Autodesk Inventor part; units mm, degrees
ref_plane "YZ Plane" through (0, 0, 0) normal (1, 0, 0) x (0, 1, 0)
ref_plane "XZ Plane" through (0, 0, 0) normal (0, 1, 0) x (-1, 0, 0)
ref_plane "XY Plane" through (0, 0, 0) normal (0, 0, 1) x (1, 0, 0)
sketch "Sketch3" plane through (0, 0, 0) normal (0, 1, 0) x (-1, 0, 0)
  circle A0 centre (0, 0) radius 5
  dimension "d8" = 10
extrude "Extrusion3" add sketch "Sketch3" along normal blind 20
sketch "Sketch4" plane through (0, 0, 0) normal (1, 0, 0) x (0, 1, 0)
  circle A0 centre (25, 0) radius 3.5
  circle A1 centre (25, 0) radius 5
  line L0 (20, -5) -> (20, 5)
  line L1 (20, -5) -> (25, -5)
  line L2 (20, 5) -> (25, 5)
  point P0 (0, 0)
  point P1 (25, 5)
  point P2 (52.9865, 4.5767)
  point P3 (20, 0)
  dimension "d11" = 7
  dimension "d12" = 10
extrude "Extrusion4" add sketch "Sketch4" along normal mid plane 3
properties part number "FP V2 Z Axis connector"
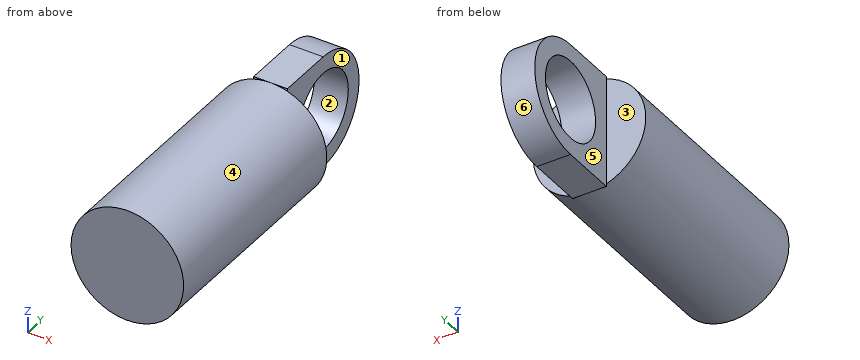
Read the model definition and answer for the solid it produces. Units are mm, in the model's axes. Face numbers are marked on the shaded views. A direction names the side the tool comes from. Give positions to 0.01 mm unless a question says otherwise; leave off trailing zeros. Loops run counter-clockwise (first coordinate to the right, second up) from the corner with the lowest first, then second, coordinate; pieces in that order, holes last.
Item 1: The part is cut by section B-B (y = 22.25). Write down the section's boundary in (x, z).
Item 2: Each of these flat-tipped pins is pushed along its axis until it touches: pin 1 Ø3 at (x, z) = (2.5, -3) entering from +Y; pin 2 Ø3 at (x, y) = (3.5, 18.5) entering from -Z; pin 3 Ø1 at (x, z) = (-3, -2) entering from +Y. Where does it stop, or does it pass through?
Item 3: The part is cut by section A-A (z = 0). Write down the section's boundary in (x, y).
Item 4: The part is cut by section C-C (z = 4). Write down the section's boundary in (x, y), and give its area (3 significant figures).
Item 5: Find the intervals of material crossed by line 1 along Z through (x, y) = (-0.85, 25); line 2 along X through (y, z) = (20.25, 3.25); line 3 along Y through (x, z) = (3, -0.75), in increasing order.
Item 6: The part is cut by section D-D (z = -3). Write down the section's boundary in (x, y), and give its area (3 significant figures).
Item 7: For the marked faces 4, 5 and 6, determine the directions among +Z, -Z, +X, -X, +Y, -Y from which every point of the face is accessible in a straight line to the end or side of a thin tool.
Item 8: The mould has two halves that part along Y. Classify the marked faces 1, 2 and 3: released by +Y, released by -Y, zero draft, split by the parting line, or undercut.
Taken from the geometry:
1. outline: (-1.5, -5) - (1.5, -5) - (1.5, -2.17) - (-1.5, -2.17) - close; (-1.5, 2.17) - (1.5, 2.17) - (1.5, 5) - (-1.5, 5) - close
2. pin 1: stops at y = 29.63
2. pin 2: stops at z = -4.58
2. pin 3: stops at y = 20
3. outline: (-5, 0) - (5, 0) - (5, 20) - (1.5, 20) - (1.5, 21.5) - (-1.5, 21.5) - (-1.5, 20) - (-5, 20) - close; (-1.5, 28.5) - (1.5, 28.5) - (1.5, 30) - (-1.5, 30) - close
4. outline: (-3, 0) - (3, 0) - (3, 20) - (1.5, 20) - (1.5, 28) - (-1.5, 28) - (-1.5, 20) - (-3, 20) - close
4. area: 144 mm2
5. line 1: z = -5 to -3.5, 3.5 to 5
5. line 2: x = -1.5 to 1.5
5. line 3: y = 0 to 20
6. outline: (-4, 0) - (4, 0) - (4, 20) - (1.5, 20) - (1.5, 23.2) - (-1.5, 23.2) - (-1.5, 20) - (-4, 20) - close; (-1.5, 26.8) - (1.5, 26.8) - (1.5, 29) - (-1.5, 29) - close
6. area: 176 mm2
7. face 4: -Y
7. face 5: +Z, -Z, -X, +Y
7. face 6: +X, -X, +Y
8. face 1: zero draft
8. face 2: undercut
8. face 3: released by +Y
